Verification items for the finished model (mm, model axes). Coordinates: 2 decimals unless noted, no trailing zeros. Write each loop counter-clockwise with the first axis right and the second up, starting at its lowest first coordinate (ties: lowest second). Pieces come first, ordered by that corner, then holes. Notation, with made-up numbers: (69, 48) -> (90, 48) arc R19 ccw to (90, 70) -> close; hole circle Ø9 at (77, -11.5). An arc over 180 degrees is marked (long way). Answer in a Markdown table with one row per item.
```python
from build123d import *

# Parameters (mm, degrees)
SKETCH_1_R          = 2.5
EXTRUDE_1_DEPTH     = 4
SKETCH_2_R          = 1
CUT_EXTRUDE_1_DEPTH = 10


with BuildPart() as part:
    # Эскиз1 → Бобышка-Вытянуть1 (new body)
    with BuildSketch(Plane(origin=(0, 0, 0), x_dir=(0, 0, -1), z_dir=(1, 0, 0))):
        Polygon((40, 15), (20, 35), (20, 90), (0, 90), (0, 0), (40, 0), align=None)
        with Locations((15, 10)):
            Circle(SKETCH_1_R, mode=Mode.SUBTRACT)
        with Locations((35, 10)):
            Circle(SKETCH_1_R, mode=Mode.SUBTRACT)
    extrude(amount=EXTRUDE_1_DEPTH)

    # Эскиз2 → Вырез-Вытянуть1 (cut)
    with BuildSketch(Plane(origin=(4, 0, 0), x_dir=(0, 0, -1), z_dir=(1, 0, 0))):
        with Locations((0.5, 2)):
            Circle(SKETCH_2_R)
        with Locations((0.5, 6)):
            Circle(SKETCH_2_R)
        with Locations((0.5, 10)):
            Circle(SKETCH_2_R)
        with Locations((0.5, 14)):
            Circle(SKETCH_2_R)
        with Locations((0.5, 18)):
            Circle(SKETCH_2_R)
        with Locations((0.5, 22)):
            Circle(SKETCH_2_R)
        with Locations((0.5, 26)):
            Circle(SKETCH_2_R)
        with Locations((0.5, 30)):
            Circle(SKETCH_2_R)
        with Locations((0.5, 34)):
            Circle(SKETCH_2_R)
        with Locations((0.5, 38)):
            Circle(SKETCH_2_R)
        with Locations((0.5, 42)):
            Circle(SKETCH_2_R)
        with Locations((0.5, 46)):
            Circle(SKETCH_2_R)
        with Locations((0.5, 50)):
            Circle(SKETCH_2_R)
        with Locations((0.5, 54)):
            Circle(SKETCH_2_R)
        with Locations((0.5, 58)):
            Circle(SKETCH_2_R)
        with Locations((0.5, 62)):
            Circle(SKETCH_2_R)
        with Locations((0.5, 66)):
            Circle(SKETCH_2_R)
        with Locations((0.5, 70)):
            Circle(SKETCH_2_R)
        with Locations((0.5, 74)):
            Circle(SKETCH_2_R)
        with Locations((0.5, 78)):
            Circle(SKETCH_2_R)
        with Locations((0.5, 82)):
            Circle(SKETCH_2_R)
        with Locations((0.5, 86)):
            Circle(SKETCH_2_R)
    extrude(amount=-CUT_EXTRUDE_1_DEPTH, mode=Mode.SUBTRACT)


solid = part.part
```
1. Release check for a two-part mould opening along Y. For faces 1 (the face through (2, 40, 0)), 2 (the face through (2, 0, -20)), 3 (the face through (2, 74, -1.5)) record: released by +Y, released by -Y, zero draft, split by the parting line, or undercut.
Findings below:
| item | result |
|---|---|
| face 1 | zero draft |
| face 2 | released by -Y |
| face 3 | undercut |
2. Sectioned sample at B-B, the plane z = -35. Record the cut outline in (x, y), and give its area (3 significant figures).
Findings below:
| item | result |
|---|---|
| outline | (0, 0) -> (4, 0) -> (4, 7.5) -> (0, 7.5) -> close; (0, 12.5) -> (4, 12.5) -> (4, 20) -> (0, 20) -> close |
| area | 60.0 mm² |
3. Material ranges on probe 1 along Z at (x, y) = (1.6, 58); probe 2 along Z at (x, y) = (0.5, 44); probe 3 along Y at (x, z) = (2.5, -32), recorded low to high. Write a range as from..to.
Findings below:
| item | result |
|---|---|
| probe 1 | z = -20..-1.5 |
| probe 2 | z = -20..0 |
| probe 3 | y = 0..23 |
4. Sectioned sample at D-D, the plane y = 6. Record the cut outline in (x, z), and give its area (3 significant figures).
Findings below:
| item | result |
|---|---|
| outline | (0, -40) -> (4, -40) -> (4, -1.5) -> (0, -1.5) -> close |
| area | 154 mm² |
5. Sectioned sample at C-C, the plane x = 1.15. Count the separate pieces of the cut face and the enclosed holes in it, and give its area (3 significant figures).
Findings below:
| item | result |
|---|---|
| separate pieces | 1 |
| enclosed holes | 2 |
| area | 2,210 mm² |
6. Go/stop test with a flat-tipped pin: pin 1 (1.2 mm diameter, centred on y = 74, z = -0.5, fed in from -X). Record where the tip stops, or that it passes through.
Findings below:
| item | result |
|---|---|
| pin 1 | passes through |
7. Sectioned sample at A-A, the plane z = -15. Record the cut outline in (x, y), and give its area (3 significant figures).
Findings below:
| item | result |
|---|---|
| outline | (0, 0) -> (4, 0) -> (4, 7.5) -> (0, 7.5) -> close; (0, 12.5) -> (4, 12.5) -> (4, 90) -> (0, 90) -> close |
| area | 340 mm² |
